Source: CAD feature listing. Evaluate the final solid. Frame: model axes, mm. Round coordinates to 2 decimals unless told otherwise and drop trailing zeros. Order: outer loops, then holes, each group sorted by start corner. A loop starts at its lowest first (then second) coordinate and runs counter-clockwise, first axis right, second up. Notation, with made-up numbers: (46.25, 44) -> (71.25, 44) arc R24 ccw to (71.25, 55) -> close; hole circle Ø9 at (10.5, 13.5). An arc over 180 degrees is marked (long way). Answer as CSV lines item,"result".
Autodesk Inventor part; units mm, degrees
ref_plane "YZ Plane" through (0, 0, 0) normal (1, 0, 0) x (0, 1, 0)
ref_plane "XZ Plane" through (0, 0, 0) normal (0, 1, 0) x (-1, 0, 0)
ref_plane "XY Plane" through (0, 0, 0) normal (0, 0, 1) x (1, 0, 0)
sketch "スケッチ1" plane through (0, 0, 0) normal (0, 0, 1) x (1, 0, 0)
  circle A0 centre (96.1098, 17.5902) radius 9.025 construction
  circle A1 centre (128.7687, 16.8502) radius 6.025 construction
  line L0 (78.0196, 48.6804) -> (110.2, 48.6804) construction
  line L1 (127.2, -14.5) -> (65.0196, -14.5)
  line L2 (65.0196, -14.5) -> (65.0196, 33.6804) construction
  circle A2 centre (96.1098, 17.5902) radius 5.0587 construction
  circle A3 centre (128.7687, 16.8502) radius 29.3819 construction
  circle A4 centre (128.7687, 16.8502) radius 31.3502
  arc A5 (102.5247, 30.0621) -> (101.9533, 4.8405) centre (96.1098, 17.5902) ccw
  line L3 (88.0848, 48.6804) -> (121.9521, 48.6804)
  arc A6 (133.1613, 47.8912) -> (121.9521, 48.6804) centre (121.9521, -31.3196) ccw
  arc A7 (88.0848, 48.6804) -> (82.0848, 42.6804) centre (88.0848, 42.6804) ccw
  line L4 (82.0848, 42.6804) -> (82.0848, -14.5)
  circle A8 centre (96.1098, 17.5902) radius 4.025
  circle A9 centre (128.7687, 16.8502) radius 4.025
  line L5 (127.2, -14.5) -> (128.7687, -14.5)
  circle A10 centre (68.0196, 17.5902) radius 1.5
  circle A11 centre (96.1098, 45.6804) radius 1.5
  circle A12 centre (74.3628, 28.0235) radius 1.3
  circle A13 centre (85.6765, 39.3372) radius 1.3
  circle A14 centre (106.5431, 39.3372) radius 1.3
  circle A15 centre (117.8569, 28.0235) radius 1.3
  circle A16 centre (117.8569, 7.1569) radius 1.3
  circle A17 centre (106.5431, -4.1569) radius 1.3
  circle A18 centre (85.6765, -4.1569) radius 1.3
  circle A19 centre (74.3628, 7.1569) radius 1.3
  point P0 (0, 0)
  point P1 (0, 0)
  point P2 (80.0196, 33.6804)
  dimension "d0" = 5
  dimension "d1" = 80
  dimension "d2" = 6
  dimension "d3" = 8.05
  dimension "d4" = 8.05
  dimension "d7" = 3
  dimension "d8" = 3
  dimension "d9" = 2.6
  dimension "d10" = 16
extrude "押し出し1" add sketch "スケッチ1" along normal blind 3 contours L1 L4 A5 A4 A17 L5 | A4 A17 A8 A14 | L4 A7 L3 A6 A4 A14 A5 | A5 A4 A8
properties part number "外側フレーム" material "アルミニウム 2014-T4"
1. Line query: L1, parallel to X at y = 16, z = 2.2; L2, parallel to X at y = 15, z = 2.45; L3, parallel to X at y = 28.5, z = 2.7. Output: solid intervals per line, ascending. Write a range as [from, to].
Results below:
L1,"[82.08, 92.41], [99.81, 124.83], [132.7, 160.11]"
L2,"[82.08, 93.03], [99.19, 125.19], [132.34, 160.06]"
L3,"[82.08, 116.65], [119.07, 157.87]"
2. Section query B-B on z = 0.7. Give the number of separate pieces and of enclosed holes in the cut face, and give its area (3 significant figures).
Results below:
separate pieces,"1"
enclosed holes,"9"
area,"4,340 mm2"
3. Pin query (flat end, axial travel): pin 1 (3.5 mm diameter, centred on x = 117.86, y = 7.16, fed in from +Z); pin 2 (1 mm diameter, centred on y = -6.5, z = 0.5, fed in from +X); pin 3 (1 mm diameter, centred on x = 147, z = 1.5, fed in from -Y). Return the tip coordinate at first contact, or that it passes through.
Results below:
pin 1,"z = 3"
pin 2,"x = 150.23"
pin 3,"y = -9"
4. Section query D-D on y = 0.5. Return loops of the section in (x, z).
Results below:
outline,"(82.08, 0) -> (155.52, 0) -> (155.52, 3) -> (82.08, 3) -> close"
5. Section query A-A on x = 126.5. Return loops of the section in (y, z).
Results below:
outline,"(-14.5, 0) -> (13.53, 0) -> (13.53, 3) -> (-14.5, 3) -> close; (20.17, 0) -> (48.55, 0) -> (48.55, 3) -> (20.17, 3) -> close"
6. Mould query, pull axis Y, two halves, no side actions, for faces 1 (the flat face through (106, -14.5, 1)), 2 (the cylindrical face through (124.748, 16.673, 1.479)), 3 (the cylindrical face through (83.8, 46.88, 1.48)), 4 (the cylindrical face through (116.899, 27.145, 1.479)). Classes: released by +Y, released by -Y, zero draft, split by the parting line, or undercut.
Results below:
face 1,"released by -Y"
face 2,"undercut"
face 3,"released by +Y"
face 4,"undercut"
7. Section query C-C on x = 96.5. Return loops of the section in (y, z).
Results below:
outline,"(-14.5, 0) -> (13.58, 0) -> (13.58, 3) -> (-14.5, 3) -> close; (21.6, 0) -> (44.23, 0) -> (44.23, 3) -> (21.6, 3) -> close; (47.13, 0) -> (48.68, 0) -> (48.68, 3) -> (47.13, 3) -> close"
